from build123d import *

# Parameters (mm, degrees)
BOSS_EXTRU_1_DEPTH      = 6
ESQUISSE3_R             = 4.5
ESQUISSE3_R_2           = 1.6
ENL_V_MAT_EXTRU_1_DEPTH = 7
ENL_V_MAT_EXTRU_2_DEPTH = 4
CONG_1_R                = 1


with BuildPart() as part:
    # Esquisse1 → Boss.-Extru.1 (new body)
    with BuildSketch(Plane.XY):
        with BuildLine():
            Line((-27.254178511, 7), (-13.254178511, 7))
            ThreePointArc((-13.254178511, 7), (-6.254178511, 0), (-13.254178511, -7))
            Line((-13.254178511, -7), (-27.254178511, -7))
            ThreePointArc((-27.254178511, -7), (-34.254178511, 0), (-27.254178511, 7))
        make_face()
    extrude(amount=BOSS_EXTRU_1_DEPTH)

    # Esquisse3 → Enlèv. mat.-Extru.1 (cut, through all)
    with BuildSketch(Plane.XY.offset(6)):
        with Locations((-20.254178511, 0)):
            Circle(ESQUISSE3_R)
        with Locations((-30.254178511, 0)):
            Circle(ESQUISSE3_R_2)
        with Locations((-10.254178511, 0)):
            Circle(ESQUISSE3_R_2)
    extrude(amount=-ENL_V_MAT_EXTRU_1_DEPTH, mode=Mode.SUBTRACT)

    # Esquisse4 → Enlèv. mat.-Extru.2 (cut)
    with BuildSketch(Plane.XY.offset(6)):
        Polygon((-13.754178511, -3.75277675), (-13.754178511, 3.75277675), (-20.254178511, 7.505553499), (-26.754178511, 3.75277675), (-26.754178511, -3.75277675), (-20.254178511, -7.505553499), align=None)
    extrude(amount=-ENL_V_MAT_EXTRU_2_DEPTH, mode=Mode.SUBTRACT)

    # Congé1
    cong_1_edges = [part.edges().sort_by_distance(p)[0] for p in [
        (-6.254178511, 0, 6),
        (-16.316356337, 7, 6),
        (-16.316356337, -7, 6),
        (-24.192000685, 7, 6),
        (-19.378534164, -7, 4),
        (-21.129822858, -7, 4),
        (-21.129822858, 7, 4),
        (-19.378534164, 7, 4),
        (-34.254178511, 0, 6),
        (-20.254178511, 7, 0),
        (-6.254178511, 0, 0),
        (-20.254178511, -7, 0),
        (-34.254178511, 0, 0),
        (-24.192000685, -7, 6),
    ]]
    fillet(cong_1_edges, radius=CONG_1_R)


solid = part.part
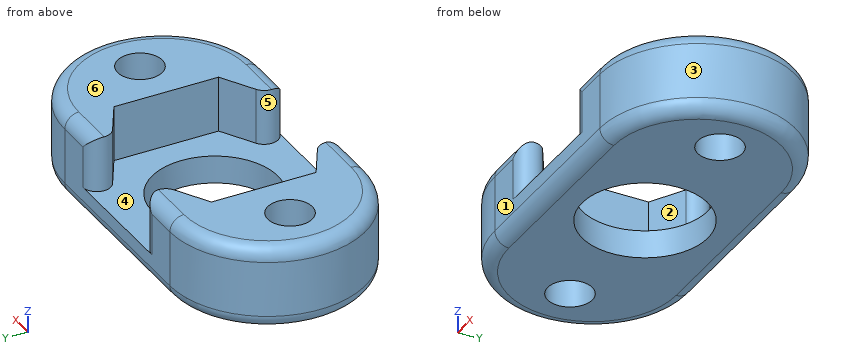
Source: CAD feature listing. Evaluate the final solid. Frame: model axes, mm. Face numbers are marked on the shaded views. A direction names the side the tool comes from. Round coordinates to 2 decimals unless told otherwise and drop trailing zeros. Order: outer loops, then holes, each group sorted by start corner. A loop starts at its lowest first (then second) coordinate and runs counter-clockwise, first axis right, second up. Notation, with made-up numbers: (28.5, -11.75) - (71.5, -11.75) arc R25 cw to (71.5, 22.25) - close; hole circle Ø3 at (-6, 64.5). An arc over 180 degrees is marked (long way). Use a Markdown table: item, result. Add a question column.
1. Section query D-D (x = -14.75). Return the cut outline in (y, z).
2. Set-up query: the marked faces 5 and 6. Return all of +Z, -Z, +X, -X, +Y, -Y with unobstructed straight access to the full face (end or side cutting, diameter ignored); none if empty.
3. Section query C-C (y = 0). Return the cut outline in (x, z), then the cut area to 3 significant figures.
4. Section query B-B (z = 5.55). Return the cut outline in (x, y).
5. Line query: probe 1 along X at (y, z) = (0.5, 3.4); probe 2 along X at (y, z) = (1.25, 1.8); probe 3 along Y at (x, z) = (-25, 2.3). Output: solid intervals per line, ascending.
6. Mould query, pull axis X, two halves, no side actions, for the marked faces 1, 2, 3 and 4. Classes: +X half, -X half, draft (parallel to the pull), parting line (faces both ways), or undercut.
7. Section query A-A (x = -20.25). Return the cut outline in (y, z).
8. First-contact query: pin 1 (1.2 mm diameter, centred on y = 1, z = 4.5, fed in from -X); pin 2 (1.2 mm diameter, centred on y = 1.5, z = 4, fed in from +X); pin 3 (4 mm diameter, centred on x = -21, y = 2.5, fed in from +Z). Flat tips, straight axial feed; report the tip coordinate or a pass-through.
Derived:
| question | item | result |
|---|---|---|
| 1 | outline | (-7, 1) arc R1 ccw to (-6, 0) - (6, 0) arc R1 ccw to (7, 1) - (7, 5) arc R1 ccw to (6, 6) - (4.33, 6) - (4.33, 2) - (-4.33, 2) - (-4.33, 6) - (-6, 6) arc R1 ccw to (-7, 5) - close |
| 2 | face 5 | +Z |
| 2 | face 6 | +Z, +X, -X, +Y, -Y |
| 3 | outline | (-34.25, 1) arc R1 ccw to (-33.25, 0) - (-31.85, 0) - (-31.85, 6) - (-33.25, 6) arc R1 ccw to (-34.25, 5) - close; (-28.65, 0) - (-24.75, 0) - (-24.75, 2) - (-26.75, 2) - (-26.75, 6) - (-28.65, 6) - close; (-15.75, 0) - (-11.85, 0) - (-11.85, 6) - (-13.75, 6) - (-13.75, 2) - (-15.75, 2) - close; (-8.65, 0) - (-7.25, 0) arc R1 ccw to (-6.25, 1) - (-6.25, 5) arc R1 ccw to (-7.25, 6) - (-8.65, 6) - close |
| 3 | area | 58.7 mm2 |
| 4 | outline | (-27.25, -6.84) - (-24.31, -6.84) arc R1 ccw to (-24.36, -5.13) - (-26.75, -3.75) - (-26.75, 3.75) - (-24.36, 5.13) arc R1 ccw to (-24.31, 6.84) - (-27.25, 6.84) arc R6.84 ccw to start; (-16.2, -6.84) - (-13.25, -6.84) arc R6.84 ccw to (-13.25, 6.84) - (-16.2, 6.84) arc R1 ccw to (-16.15, 5.13) - (-13.75, 3.75) - (-13.75, -3.75) - (-16.15, -5.13) arc R1 ccw to start; hole circle Ø3.2 at (-30.25, 0); hole circle Ø3.2 at (-10.25, 0) |
| 5 | probe 1 | -34.24 to -31.77, -28.73 to -26.75, -13.75 to -11.77, -8.73 to -6.27 |
| 5 | probe 2 | -34.14 to -31.25, -29.26 to -24.58, -15.93 to -11.25, -9.26 to -6.37 |
| 5 | probe 3 | -7 to -4.77, 4.77 to 7 |
| 6 | face 1 | draft |
| 6 | face 2 | undercut |
| 6 | face 3 | +X half |
| 6 | face 4 | undercut |
| 7 | outline | (-7, 1) arc R1 ccw to (-6, 0) - (-4.5, 0) - (-4.5, 2) - (-7, 2) - close; (4.5, 0) - (6, 0) arc R1 ccw to (7, 1) - (7, 2) - (4.5, 2) - close |
| 8 | pin 1 | x = -34.24 |
| 8 | pin 2 | x = -6.31 |
| 8 | pin 3 | z = 2 |
